Part print with two shaded views. Sizes in mm from the minimum x, y, z corner. A direction names the side the tool comes from. Coordinates: 2 decimals unless noted, no trailing zeros. Loops run counter-clockwise (first coordinate to the right, second up) from the corner with the lowest first, then second, coordinate; pieces in that order, holes last. Notation, with made-up numbers: (77, -3.75) -> (92, -3.75) arc R7 cw to (92, 7.25) -> close; hole circle Ø6 at (38.25, -3.5). An arc over 180 degrees is marked (long way). Use one line per item in the form item = value.
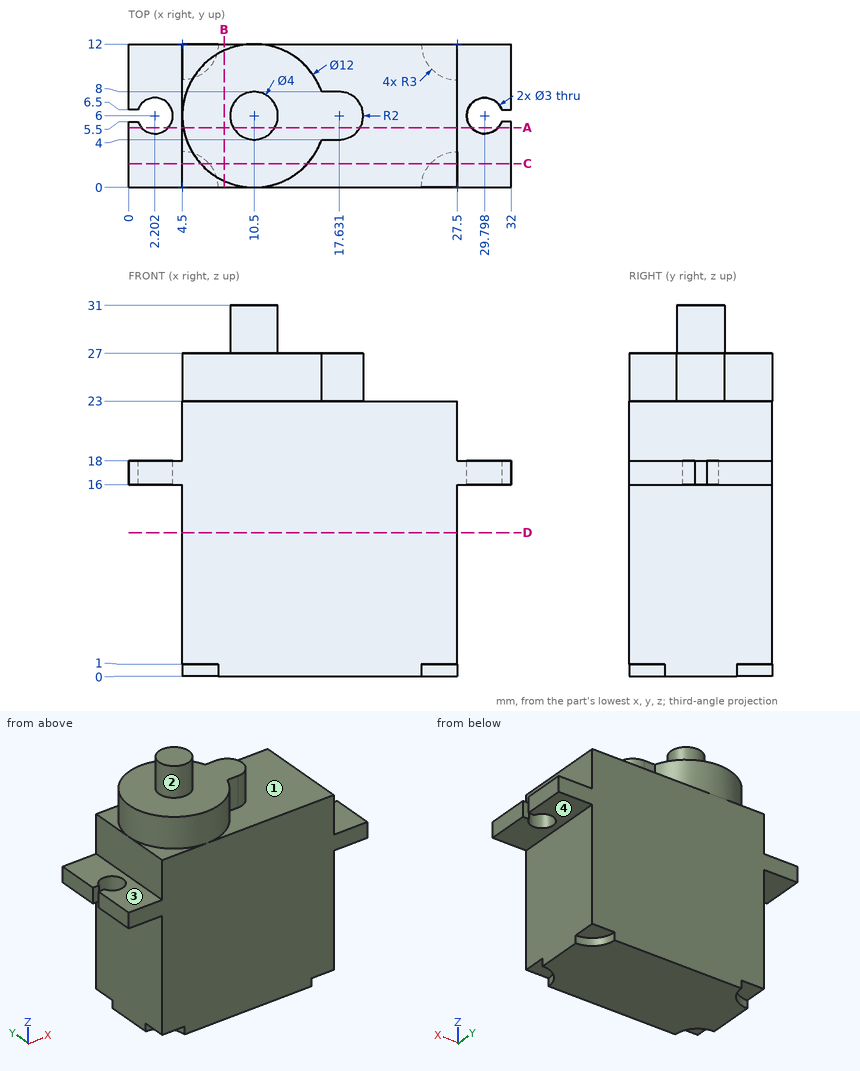
Q1. Which spindle directions (+Z, -Z, +X, -X, +Y, -Y) get a long thin tool onto all of the face, cutting with end or side? Do the marked faces 1, 2, 3 and 4. Say none if no direction does.
Result:
face_1 = +Z, +X
face_2 = +Z
face_3 = +Z, -X, +Y, -Y
face_4 = -Z, +X, +Y, -Y
Q2. Pin check, flat tips, straight feed: pin 1 Ø0.9 at (x, y) = (26, 10.5) entering from -Z; pin 2 Ø6 at (x, y) = (19, 5) entering from +Z; pin 3 Ø5.5 at (y, z) = (6.5, 21) entering from -X. Stop position of each tip, or through.
Result:
pin_1 = 1
pin_2 = 27
pin_3 = 4.5
Q3. Band-saw the part on D-D, the plane z = 12. Write the cut outline in (x, y), and give its area (3 significant figures).
Result:
outline = (4.5, 0) -> (27.5, 0) -> (27.5, 12) -> (4.5, 12) -> close
area = 276 mm2
Q4. Band-saw the part on A-A, the plane y = 5. State how many separate pieces and enclosed holes the cut face has, and give its area (3 significant figures).
Result:
separate_pieces = 3
enclosed_holes = 0
area = 611 mm2
Q5. Band-saw the part on C-C, the plane y = 2. Write the cut outline in (x, z), and give its area (3 significant figures).
Result:
outline = (0, 16) -> (4.5, 16) -> (4.5, 1) -> (6.74, 1) -> (6.74, 0) -> (25.26, 0) -> (25.26, 1) -> (27.5, 1) -> (27.5, 16) -> (32, 16) -> (32, 18) -> (27.5, 18) -> (27.5, 23) -> (14.97, 23) -> (14.97, 27) -> (6.03, 27) -> (6.03, 23) -> (4.5, 23) -> (4.5, 18) -> (0, 18) -> close
area = 578 mm2
Q6. Band-saw the part on B-B, the plane x = 8. Write the cut outline in (y, z) (1 decimal), and give its area (3 significant figures).
Result:
outline = (0, 0) -> (12, 0) -> (12, 23) -> (11.5, 23) -> (11.5, 27) -> (0.5, 27) -> (0.5, 23) -> (0, 23) -> close
area = 320 mm2
Q7. Wall check: line 1 along X through (y, z) = (5, 17) (1 decimal); line 2 along X through (y, z) = (2, 13.5); line 3 along X through (y, z) = (6, 17.4). Give the ranges that are in metal, low to high.
Result:
line_1 = 0 to 1.1, 3.3 to 28.7, 30.9 to 32
line_2 = 4.5 to 27.5
line_3 = 3.7 to 28.3
